The listing builds one solid part. Answer for the finished solid, in the listing's coordinates (mm). A direction names the side the tool comes from. Round coordinates to 2 decimals unless told otherwise and drop trailing zeros. Write each loop counter-clockwise with the first axis right and the second up, starting at its lowest first coordinate (ties: lowest second). Pieces come first, ordered by that corner, then holes. Notation, with made-up numbers: M 85,-14.5 L 100,-14.5 A37 ccw 100,24.5 Z; hole C 60,74 d7. An arc over 180 degrees is marked long. One line per item, written item: value. Start each with the question number.
(1) Given P1, Ø9, axis at x = -19.5, y = -8, coming from the -Z side; P2, Ø6, axis at x = 1.5, y = 1, coming from the +Z side; P3, Ø5, axis at x = 1.5, y = -12, coming from the +Z side; P4, Ø2, axis at x = -3, z = -16, coming from the +Y side, each flat-ended and moving along its own axis, determine where each tip first touches the part or whether it passes through.
(2) Section C-C (y = -7.5) is taken. Determine the outline of the cut face in (x, z), plus the area to 3 significant figures.
(3) For a pull along Y with two mould halves and no side action, classify faces 6 (the flat face through (4.59, -9.07, 2.46)), 7 (the flat face through (4.516, -10.457, 2.465)), 8 (the flat face through (-11.38, -0.05, 2.46)), 9 (the flat face through (2.3, -2.3, 11)) as released by +Y, released by -Y, zero draft, split by the parting line, or undercut.
(4) For faces 1 (the flat face through (-11.2, -18.41, 2.46)), 2 (the cylindrical face through (7.136, -14.358, 2.465)), 3 (the cylindrical face through (-15.85, 0.75, 2.46)), 4 (the flat face through (-5, -9, 0)), 5 (the cylindrical face through (5.198, 1.637, 8.141)), determine the directions among +Z, -Z, +X, -X, +Y, -Y from which every point of the face is accessible in a straight line to the end or side of a thin tool.
(5) Consider probe 1 along Z at (x, y) = (5.5, -0.5); probe 2 along Z at (x, y) = (-10, -18.5); probe 3 along Y at (x, z) = (2, 6). Determine where each line is inside the solid, lowest interval first.
(6) Section B-B (x = -18) is taken. Determine the outline of the cut face in (y, z), plus the area to 3 significant figures.
(7) Section D-D (z = -25) is taken. Determine the outline of the cut face in (x, y).
```python
from build123d import *

# Parameters (mm, degrees)
SKETCH1_R           = 6.5
BOSS_EXTRUDE1_DEPTH = 11
SKETCH2_R           = 2.75
CUT_EXTRUDE1_DEPTH  = 3
SKETCH3_OUTSIDE_W   = 19.284
SKETCH3_OUTSIDE_H   = 19.284
SKETCH3_OUTSIDE_R   = 5.45
CUT_EXTRUDE2_DEPTH  = 5.8
SKETCH4_R           = 3.5
BOSS_EXTRUDE2_DEPTH = 40
JOIN2_OUTLINE_R     = 5.75
JOIN2_OUTLINE_R_2   = 6.5
JOIN2_DEPTH         = 5
JOIN2_START         = -2
JOIN2_2_OUTLINE_R   = 5.75
JOIN2_2_DEPTH       = 4


# Read off the part's stored shape, not the designer's step: Join2
with BuildPart() as part:
    # Sketch1 → Boss-Extrude1 (new body)
    with BuildSketch(Plane.XY):
        Circle(SKETCH1_R)
    extrude(amount=BOSS_EXTRUDE1_DEPTH)

    # Sketch2 → Cut-Extrude1 (cut)
    with BuildSketch(Plane.XY.offset(11)):
        Circle(SKETCH2_R)
    extrude(amount=-CUT_EXTRUDE1_DEPTH, mode=Mode.SUBTRACT)

    # Sketch3 outside → Cut-Extrude2 (cut)
    with BuildSketch(Plane.XY.offset(11)):
        Rectangle(SKETCH3_OUTSIDE_W, SKETCH3_OUTSIDE_H)
        Circle(SKETCH3_OUTSIDE_R, mode=Mode.SUBTRACT)
    extrude(amount=-CUT_EXTRUDE2_DEPTH, mode=Mode.SUBTRACT)

    # Sketch4 → Boss-Extrude2 (add)
    with BuildSketch(Plane(origin=(0, 0, 0), x_dir=(-1, 0, 0), z_dir=(0, 0, -1))):
        Circle(SKETCH4_R)
    extrude(amount=BOSS_EXTRUDE2_DEPTH)

    # Join2 outline → Join2 (add)
    with BuildSketch(Plane.XY):
        with BuildLine():
            Line((4.091169505, -11.107165908), (4.953212207, -9.78769749))
            Line((4.953212207, -9.78769749), (4.215242705, -8.329447379))
            ThreePointArc((4.215242705, -8.329447379), (8.329447379, 4.215242705), (-4.215242705, 8.329447379))
            Line((-4.215242705, 8.329447379), (-4.56983635, 8.149999907))
            ThreePointArc((-4.56983635, 8.149999907), (-7.929245952, 4.942970907), (-9.329576894, 0.51468217))
            Line((-9.329576894, 0.51468217), (-10.953000775, 0.604241143))
            Line((-10.953000775, 0.604241143), (-11.815043478, -0.715227275))
            ThreePointArc((-11.815043478, -0.715227275), (-15.913949613, 0.756712749), (-20.236162848, 0.221818664))
            Line((-20.236162848, 0.221818664), (-21.168032047, -0.249767825))
            ThreePointArc((-21.168032047, -0.249767825), (-25.282236722, -12.794457909), (-12.737546638, -16.908662583))
            Line((-12.737546638, -16.908662583), (-11.999577135, -18.366912694))
            Line((-11.999577135, -18.366912694), (-10.376153254, -18.456471667))
            ThreePointArc((-10.376153254, -18.456471667), (-1.56125853, -28.300730731), (8.283000534, -19.485836007))
            Line((8.283000534, -19.485836007), (8.336201554, -18.521468017))
            ThreePointArc((8.336201554, -18.521468017), (7.105378721, -14.303781228), (4.091169505, -11.107165908))
        make_face()
        with Locations((-1.04657636, -18.971153837)):
            Circle(JOIN2_OUTLINE_R, mode=Mode.SUBTRACT)
        with Locations((-16.952789342, -8.579215204)):
            Circle(JOIN2_OUTLINE_R, mode=Mode.SUBTRACT)
        Circle(JOIN2_OUTLINE_R_2, mode=Mode.SUBTRACT)
    extrude(amount=JOIN2_DEPTH)

    # Join2 2 outline → Join2 2 (add)
    with BuildSketch(Plane.XY.offset(JOIN2_START)):
        with Locations((-1.04657636, -18.971153837)):
            Circle(JOIN2_2_OUTLINE_R)
        with Locations((-16.952789342, -8.579215204)):
            Circle(JOIN2_2_OUTLINE_R)
    extrude(amount=JOIN2_2_DEPTH)


solid = part.part
```
Recorded:
1. P1: stops at z = -2
1. P2: stops at z = 11
1. P3: stops at z = 5
1. P4: stops at y = 2.87
2. outline: M -26.23,0 L -22.6,0 L -22.6,-2 L -11.3,-2 L -11.3,0 L 5.56,0 L 5.56,5 L -11.3,5 L -11.3,2 L -22.6,2 L -22.6,5 L -26.23,5 Z
2. area: 148 mm2
3. face 6: undercut
3. face 7: undercut
3. face 8: released by +Y
3. face 9: zero draft
4. face 1: +Z, -Z, -X, -Y
4. face 2: +Z, -Z, +X
4. face 3: +Z, -Z, +Y
4. face 4: -Z
4. face 5: +Z
5. probe 1: z = 0 to 5.2
5. probe 2: z = 0 to 5
5. probe 3: y = -5.07 to 5.07
6. outline: M -17.86,0 L -14.23,0 L -14.23,-2 L -2.93,-2 L -2.93,0 L 0.76,0 L 0.76,5 L -2.93,5 L -2.93,2 L -14.23,2 L -14.23,5 L -17.86,5 Z
6. area: 81.7 mm2
7. outline: C 0,0 d7
